Verification items for the finished model (mm, model axes). Round coordinates to 2 decimals unless told otherwise and drop trailing zeros. Order: outer loops, then holes, each group sorted by start corner. A loop starts at its lowest first (then second) coordinate and runs counter-clockwise, first axis right, second up. Notation, with made-up numbers: (12.25, -35) -> (35.25, -35) arc R15 ccw to (35.25, -15) -> close; hole circle Ø3 at (60, 46). An arc over 180 degrees is marked (long way). Return JSON: item names as keys, results as strings. Group by question number.
Item 1: Scan lines: probe 1 along X at (y, z) = (-9.5, 1.25); probe 2 along X at (y, z) = (-28.5, 0.1); probe 3 along Y at (x, z) = (12.5, 1.45). Record each from-to range of solid material in increasing order. Write a range as from..to.
Item 2: Sectioned sample at A-A on y = 0. Record the cut outline in (x, z).
Item 3: Depth check by flat-ended pin: pin 1 Ø1.5 at (x, z) = (12.5, -1) entering from -Y; pin 2 Ø6 at (x, y) = (0, 0) entering from -Z. Enter the tip coordinate at first touch or a pass-through.
Item 4: Sectioned sample at C-C on z = -0.3. Give the number of separate pieces and of enclosed holes in the cut face, plus the area to 3 significant figures.
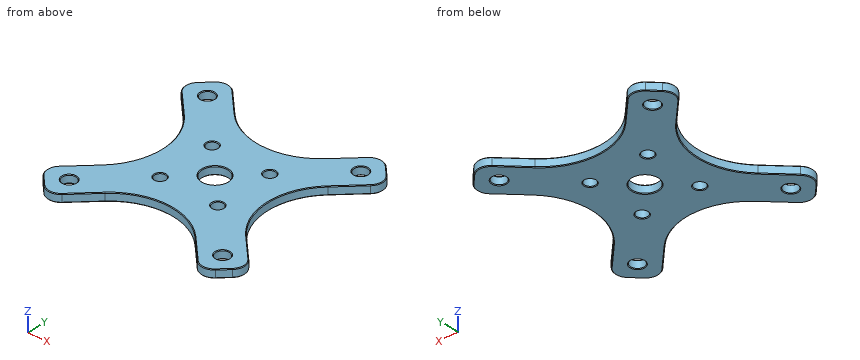
```python
from build123d import *

# Parameters (mm, degrees)
SKETCH1_R            = 5
BOSS_EXTRUDE1_DEPTH  = 1.5875
M4_CLEARANCE_HOLE1_D = 4.3
M5_CLEARANCE_HOLE1_D = 5.3
FILLET1_R            = 25
FILLET2_R            = 5
CHAMFER1_SIZE        = 0.25


with BuildPart() as part:
    # Sketch1 → Boss-Extrude1 (new, symmetric)
    with BuildSketch(Plane.XY):
        Polygon((0, 10.606601718), (30.0520382, 40.658639918), (40.658639918, 30.0520382), (10.606601718, 0), (40.658639918, -30.0520382), (30.0520382, -40.658639918), (0, -10.606601718), (-30.0520382, -40.658639918), (-40.658639918, -30.0520382), (-10.606601718, 0), (-40.658639918, 30.0520382), (-30.0520382, 40.658639918), align=None)
        Circle(SKETCH1_R, mode=Mode.SUBTRACT)
    extrude(amount=BOSS_EXTRUDE1_DEPTH, both=True)

    # M4 Clearance Hole1 (through all)
    with Locations(Plane.XY.offset(1.5875)):
        with Locations((-11.313708499, 11.313708499), (11.313708499, 11.313708499), (11.313708499, -11.313708499), (-11.313708499, -11.313708499)):
            Hole(M4_CLEARANCE_HOLE1_D / 2)

    # M5 Clearance Hole1 (through all)
    with Locations(Plane(origin=(0, 0, -1.5875), x_dir=(-1, 0, 0), z_dir=(0, 0, -1))):
        with Locations((-30.0520382, 30.0520382), (30.0520382, 30.0520382), (30.0520382, -30.0520382), (-30.0520382, -30.0520382)):
            Hole(M5_CLEARANCE_HOLE1_D / 2)

    # Fillet1
    fillet1_edges = [part.edges().sort_by_distance(p)[0] for p in [
        (0, 10.606601718, 0),
        (10.606601718, 0, 0),
        (0, -10.606601718, 0),
        (-10.606601718, 0, 0),
    ]]
    fillet(fillet1_edges, radius=FILLET1_R)

    # Fillet2
    fillet2_edges = [part.edges().sort_by_distance(p)[0] for p in [
        (30.0520382, 40.658639918, 0),
        (40.658639918, 30.0520382, 0),
        (40.658639918, -30.0520382, 0),
        (30.0520382, -40.658639918, 0),
        (-30.0520382, -40.658639918, 0),
        (-40.658639918, -30.0520382, 0),
        (-40.658639918, 30.0520382, 0),
        (-30.0520382, 40.658639918, 0),
    ]]
    fillet(fillet2_edges, radius=FILLET2_R)

    # Chamfer1
    chamfer1_edges = [part.edges().sort_by_distance(p)[0] for p in [
        (-22.097086912, 32.70368863, -1.5875),
        (-22.097086912, 32.70368863, 1.5875),
        (-20.961940777, 0, -1.5875),
        (-20.961940777, 0, 1.5875),
        (0, -20.961940777, -1.5875),
        (0, -20.961940777, 1.5875),
        (20.961940777, 0, -1.5875),
        (20.961940777, 0, 1.5875),
        (0, 20.961940777, -1.5875),
        (0, 20.961940777, 1.5875),
        (32.70368863, -22.097086912, -1.5875),
        (32.70368863, -22.097086912, 1.5875),
        (22.097086912, 32.70368863, -1.5875),
        (35.355339059, 35.355339059, -1.5875),
        (35.355339059, -35.355339059, -1.5875),
        (-22.097086912, -32.70368863, -1.5875),
        (-35.355339059, -35.355339059, -1.5875),
        (-32.70368863, 22.097086912, -1.5875),
        (-35.355339059, 35.355339059, -1.5875),
        (38.587572106, 30.0520382, -1.5875),
        (30.0520382, 38.587572106, -1.5875),
        (-30.0520382, 38.587572106, -1.5875),
        (-38.587572106, 30.0520382, -1.5875),
        (-38.587572106, -30.0520382, -1.5875),
        (-30.0520382, -38.587572106, -1.5875),
        (30.0520382, -38.587572106, -1.5875),
        (38.587572106, -30.0520382, -1.5875),
        (35.355339059, -35.355339059, 1.5875),
        (22.097086912, 32.70368863, 1.5875),
        (-35.355339059, 35.355339059, 1.5875),
        (-32.70368863, 22.097086912, 1.5875),
        (-35.355339059, -35.355339059, 1.5875),
        (-22.097086912, -32.70368863, 1.5875),
        (35.355339059, 35.355339059, 1.5875),
        (38.587572106, 30.0520382, 1.5875),
        (30.0520382, 38.587572106, 1.5875),
        (-30.0520382, 38.587572106, 1.5875),
        (-38.587572106, 30.0520382, 1.5875),
        (-38.587572106, -30.0520382, 1.5875),
        (-30.0520382, -38.587572106, 1.5875),
        (30.0520382, -38.587572106, 1.5875),
        (38.587572106, -30.0520382, 1.5875),
        (-5, 0, -1.5875),
        (-5, 0, 1.5875),
        (-9.163708499, 11.313708499, 1.5875),
        (-9.163708499, 11.313708499, -1.5875),
        (-9.163708499, -11.313708499, 1.5875),
        (-9.163708499, -11.313708499, -1.5875),
        (13.463708499, -11.313708499, 1.5875),
        (13.463708499, -11.313708499, -1.5875),
        (13.463708499, 11.313708499, 1.5875),
        (13.463708499, 11.313708499, -1.5875),
        (27.4020382, -30.0520382, -1.5875),
        (27.4020382, -30.0520382, 1.5875),
        (-32.7020382, -30.0520382, -1.5875),
        (-32.7020382, -30.0520382, 1.5875),
        (-32.7020382, 30.0520382, -1.5875),
        (-32.7020382, 30.0520382, 1.5875),
        (27.4020382, 30.0520382, -1.5875),
        (27.4020382, 30.0520382, 1.5875),
        (-32.70368863, -22.097086912, -1.5875),
        (-32.70368863, -22.097086912, 1.5875),
        (22.097086912, -32.70368863, -1.5875),
        (22.097086912, -32.70368863, 1.5875),
        (32.70368863, 22.097086912, -1.5875),
        (32.70368863, 22.097086912, 1.5875),
    ]]
    chamfer(chamfer1_edges, length=CHAMFER1_SIZE)


solid = part.part
```
Recorded:
{
 "1": {"probe 1": "-22.84..-12.47, -10.16..10.16, 12.47..22.84", "probe 2": "-38.34..-32.2, -27.9..-17.89, 17.89..27.9, 32.2..38.34", "probe 3": "-24.18..-13.24, -9.39..9.39, 13.24..24.18"},
 "2": {"outline": "(-20.96, -1.34) -> (-20.71, -1.59) -> (-5.25, -1.59) -> (-5, -1.34) -> (-5, 1.34) -> (-5.25, 1.59) -> (-20.71, 1.59) -> (-20.96, 1.34) -> close; (5, -1.34) -> (5.25, -1.59) -> (20.71, -1.59) -> (20.96, -1.34) -> (20.96, 1.34) -> (20.71, 1.59) -> (5.25, 1.59) -> (5, 1.34) -> close"},
 "3": {"pin 1": "y = -24.76", "pin 2": "through"},
 "4": {"separate pieces": "1", "enclosed holes": "9", "area": "3,040 mm²"}
}
